Autodesk Inventor part; units mm, degrees
ref_plane "YZ Plane" through (0, 0, 0) normal (1, 0, 0) x (0, 1, 0)
ref_plane "XZ Plane" through (0, 0, 0) normal (0, 1, 0) x (-1, 0, 0)
ref_plane "XY Plane" through (0, 0, 0) normal (0, 0, 1) x (1, 0, 0)
sketch "Sketch1" plane through (0, 0, 0) normal (0, 1, 0) x (-1, 0, 0)
  line L0 (30, 45) -> (-30, 45)
  line L1 (-30, 45) -> (-30, -45)
  line L2 (-30, -45) -> (30, -45)
  line L3 (30, -45) -> (30, 45)
  line L4 (30, 45) -> (-30, -45) construction
  line L5 (-30, 45) -> (30, -45) construction
  point P0 (0, 0)
  dimension "d0" = 90
  dimension "d1" = 60
extrude "Extrusion1" add sketch "Sketch1" along normal blind 20
sketch "Sketch2" plane through (0, 0, 0) normal (0, -1, 0) x (1, 0, 0)
  line L0 (26.5, 45) -> (-26.5, 45)
  line L1 (-26.5, 45) -> (-26.5, -29)
  line L2 (-26.5, -29) -> (26.5, -29)
  line L3 (26.5, -29) -> (26.5, 45)
  line L4 (-30, 45) -> (30, 45)
  point P0 (0, 0)
  dimension "d4" = 74
  dimension "d5" = 0
  dimension "d6" = 53
  dimension "d7" = 26.5
extrude "Extrusion2" add sketch "Sketch2" along normal blind 15
sketch "Sketch3" plane through (30, 0, 45) normal (1, 0, 0) x (0, 0, -1)
  line L0 (0, 0) -> (90, 0)
  line L1 (90, 0) -> (90, 20)
  line L2 (0, 20) -> (90, 20)
  line L3 (0, 0) -> (0, 20)
  line L4 (90, 0) -> (60, 0)
  line L5 (60, 0) -> (60, 20)
  line L6 (60, 20) -> (90, 20)
  line L7 (90, 20) -> (90, 0)
  point P0 (45, 0)
  dimension "d10" = 30
extrude "Extrusion3" add sketch "Sketch3" along normal blind 16 contours L5 L2 L1 L0
mirror "Mirror1" about plane through (0, 0, 0) normal (1, 0, 0) of "Extrusion3"
shell "Shell1" thickness 1 removed faces 1 at (-10, 20, 5)
ref_plane "Work Plane1" through (0, 0, 0) normal (1, 0, 0) x (0, 1, 0)
properties part number "body_bottom"
The model under review builds one solid part; all positions refer to its coordinate system, in mm. A direction names the side the tool comes from. Round coordinates to 2 decimals unless told otherwise and drop trailing zeros. Order: outer loops, then holes, each group sorted by start corner. A loop starts at its lowest first (then second) coordinate and runs counter-clockwise, first axis right, second up. Notation, with made-up numbers: (-1, 50) - (38, 50) arc R28 ccw to (38, 69) - close; hole circle Ø4 at (-27.5, -7.75). An arc over 180 degrees is marked (long way). Use one line per item in the form item = value.
Q1. Mouldability with a two-part tool opening along Z and no side actions: class faces 1 (the flat face through (0, -14, 9)), 2 (the flat face through (1, 10, -45)), 3 (the flat face through (0, 2, 45)), 4 (the flat face through (37, 10, -16)) as pulls with the +Z half, pulls with the -Z half, needs draft (parallel to the pull), parting line crosses it, or undercut.
Response values:
face_1 = undercut
face_2 = pulls with the -Z half
face_3 = pulls with the +Z half
face_4 = undercut
Q2. To check wall thickness, follow line 1 (X direction, y = 18, z = -24.5); line 2 (X direction, y = -12, z = -26); line 3 (Z direction, x = -24.5, y = -5.5). State the ranges of each line that lie inside material, in increasing order.
Response values:
line_1 = -46 to -45, 45 to 46
line_2 = -26.5 to -25.5, 25.5 to 26.5
line_3 = -29 to -28, 44 to 45
Q3. Clearance check with flat-ended pins moving along their axes: P1, Ø12, axis at y = -5, z = 7.5, coming from the -X side; P2, Ø13, axis at x = 38.5, y = 9, coming from the +Z side; P3, Ø2, axis at x = -27, y = -7.5, coming from the -Z side. State where each tip first meets the part, or that it passes through.
Response values:
P1 = -30
P2 = -15
P3 = -29
Q4. Add section D-D on y = 11. Give the boundary of the cut face in (x, z).
Response values:
outline = (-46, -45) - (46, -45) - (46, -15) - (30, -15) - (30, 45) - (-30, 45) - (-30, -15) - (-46, -15) - close; hole (-45, -44) - (45, -44) - (45, -16) - (29, -16) - (29, 44) - (-29, 44) - (-29, -16) - (-45, -16) - close
Q5. Add section A-A on y = -3.5. Give the boundary of the cut face in (x, z).
Response values:
outline = (-26.5, -29) - (26.5, -29) - (26.5, 45) - (-26.5, 45) - close; hole (-25.5, -28) - (25.5, -28) - (25.5, 44) - (-25.5, 44) - close
Q6. Add section C-C on x = 9.5. Give the boundary of the cut face in (y, z), then the cut area to 3 significant figures.
Response values:
outline = (-15, -29) - (0, -29) - (0, -45) - (20, -45) - (20, -44) - (1, -44) - (1, -28) - (-14, -28) - (-14, 44) - (20, 44) - (20, 45) - (-15, 45) - close
area = 158 mm^2
Q7. Tool access review of faces 5 (the flat face through (-26.5, -7, 9)), 6 (the flat face through (0, 3, 44)), 7 (the flat face through (38, 10, -15)), 8 (the flat face through (0, -7, -29)): name each direction out of +Z, -Z, +X, -X, +Y, -Y from which nothing blocks a thin tool from reaching the whole face with its end or side.
Response values:
face_5 = +Z, -Z, -X, -Y
face_6 = +Y
face_7 = +Z, +X, +Y, -Y
face_8 = -Z, +X, -X, -Y
Q8. Add section B-B on z = 20. Give the boundary of the cut face in (x, y), then the cut area to 3 significant figures.
Response values:
outline = (-30, 0) - (-26.5, 0) - (-26.5, -15) - (26.5, -15) - (26.5, 0) - (30, 0) - (30, 20) - (29, 20) - (29, 1) - (25.5, 1) - (25.5, -14) - (-25.5, -14) - (-25.5, 1) - (-29, 1) - (-29, 20) - (-30, 20) - close
area = 128 mm^2
